from build123d import *

# Parameters (mm, degrees)
F1_DEPTH = 6.35
F3_DEPTH = 19.05
F4_R     = 5.08


with BuildPart() as f1:
    # F0 (on Top) → F1 (new body)
    with BuildSketch(Plane.XY):
        with BuildLine():
            Line((28.575, -19.05), (28.575, 19.05))
            Line((28.575, 19.05), (12.7, 19.05))
            ThreePointArc((12.7, 19.05), (0, 6.35), (-12.7, 19.05))
            Line((-12.7, 19.05), (-28.575, 19.05))
            Line((-28.575, 19.05), (-28.575, -19.05))
            Line((-28.575, -19.05), (28.575, -19.05))
        make_face()
    extrude(amount=F1_DEPTH)

    # F2 (on face) → F3 (join)
    with BuildSketch(Plane.XY.offset(6.35)):
        with BuildLine():
            Line((-15.875, 19.05), (-15.875, 0))
            Line((-15.875, 0), (15.875, 0))
            Line((15.875, 0), (15.875, 19.05))
            Line((15.875, 19.05), (12.7, 19.05))
            ThreePointArc((12.7, 19.05), (0, 6.35), (-12.7, 19.05))
            Line((-12.7, 19.05), (-15.875, 19.05))
        make_face()
        Polygon((-25.4, 0), (-25.4, -19.05), (-19.05, -19.05), (-19.05, -12.7), (19.05, -12.7), (19.05, -19.05), (25.4, -19.05), (25.4, 0), (15.875, 0), (-15.875, 0), align=None)
    extrude(amount=F3_DEPTH)

    # F4
    f4_edges = [f1.edges().sort_by_distance(p)[0] for p in [
        (-28.575, 19.05, 3.175),
        (28.575, 19.05, 3.175),
        (-15.875, 0, 15.875),
        (15.875, 0, 15.875),
    ]]
    fillet(f4_edges, radius=F4_R)


solid = f1.part
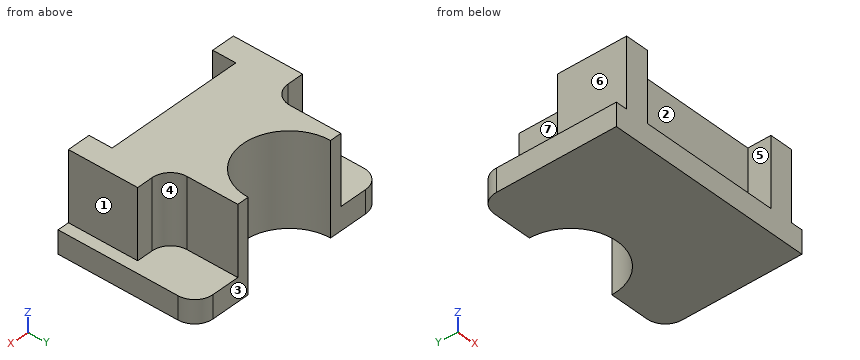
Design review of the part built by this model. Coordinates are the model's own, in mm. Face numbers are marked on the shaded views. A direction names the side the tool comes from. Give positions to 0.01 mm unless a question says otherwise; leave off trailing zeros. Write each loop counter-clockwise with the first axis right and the second up, starting at its lowest first coordinate (ties: lowest second). Pieces come first, ordered by that corner, then holes. Notation, with made-up numbers: M 21.25,22.5 L 54.25,22.5 A10 ccw 54.25,41.5 Z; hole C 15,2 d4. An arc over 180 degrees is marked long. Answer as a JSON object with one key per item and string values. Group by question number.
1) Mouldability with a two-part tool opening along X and no side actions: class the marked faces 1, 2 and 3 as released by +X, released by -X, zero draft, split by the parting line, or undercut.
2) We need section D-D (x = 22.5). Give the boundary of the cut face in (y, z).
3) Tool access review of the marked faces 4, 5, 6 and 7: name each direction out of +Z, -Z, +X, -X, +Y, -Y from which nothing blocks a thin tool from reaching the whole face with its end or side.
4) We need section B-B (z = 7.5). Give the boundary of the cut face in (x, y) (3 decimals), and give its area (3 significant figures).
5) For line 1 along X through (y, z) = (-17, 21); line 2 along Z through (x, y) = (-16.5, 9); line 3 along X through (y, z) = (-5, 7), list the stretches that pass through material, from the lowest coordinate up.
6) Clearance check with flat-ended pins moving along their axes: pin 1 Ø5 at (x, z) = (22.5, 17) entering from +Y; pin 2 Ø5 at (y, z) = (-15, 19.5) entering from +X; pin 3 Ø1.9 at (x, y) = (2.5, -17) entering from +Z. State where each tip first meets the part, or that it passes through.
7) We need section A-A (y = -5.5). Give the boundary of the cut face in (x, z) (3 decimals).
8) We need section C-C (y = 12.5). Give the boundary of the cut face in (x, z) (3 decimals), and give its area (3 significant figures).
Answer key:
{
 "1": {"face 1": "released by +X", "face 2": "undercut", "face 3": "zero draft"},
 "2": {"outline": "M -19.05,0 L 19.05,0 L 19.05,6.35 L 0,6.35 L 0,25.4 L -19.05,25.4 Z"},
 "3": {"face 4": "+Z, +X, +Y", "face 5": "+Z, -Y", "face 6": "+Z, -X, +Y, -Y", "face 7": "+Z, -X, +Y"},
 "4": {"outline": "M -25.4,-19.05 L -19.05,-19.05 L -19.05,-12.7 L 19.05,-12.7 L 19.05,-19.05 L 25.4,-19.05 L 25.4,0 L 20.955,0 A5.08 cw 15.875,5.08 L 15.875,19.05 L 12.7,19.05 A12.7 cw -12.7,19.05 L -15.875,19.05 L -15.875,5.08 A5.08 cw -20.955,0 L -25.4,0 Z", "area": "1,090 mm²"},
 "5": {"line 1": "x = -25.4 to -19.05, 19.05 to 25.4", "line 2": "z = 0 to 6.35", "line 3": "x = -25.4 to 25.4"},
 "6": {"pin 1": "stops at y = 0.09", "pin 2": "stops at x = 25.4", "pin 3": "stops at z = 6.35"},
 "7": {"outline": "M -28.575,0 L 28.575,0 L 28.575,6.35 L 25.4,6.35 L 25.4,25.4 L -25.4,25.4 L -25.4,6.35 L -28.575,6.35 Z"},
 "8": {"outline": "M -28.575,0 L -10.881,0 L -10.881,25.4 L -15.875,25.4 L -15.875,6.35 L -28.575,6.35 Z; M 10.881,0 L 28.575,0 L 28.575,6.35 L 15.875,6.35 L 15.875,25.4 L 10.881,25.4 Z", "area": "415 mm²"}
}
